```python
from build123d import *

# Parameters (mm, degrees)
BASE_FLANGE1_DEPTH            = 5
EDGE_FLANGE1_STRIP_W          = 25.2
EDGE_FLANGE1_STRIP_H          = 5
EDGE_FLANGE1_STRIP_CUT_DEPTH  = 270
EDGE_FLANGE1_RELIEF_W         = 27.7
EDGE_FLANGE1_RELIEF_H         = 2.5
EDGE_FLANGE1_RELIEF_CUT_DEPTH = 5
EDGE_FLANGE1_DEPTH            = 270
SKETCH9_R                     = 2.5
CUT_EXTRUDE1_DEPTH            = 10
FILLET1_R                     = 20
FILLET2_R                     = 2


# Sheet-metal steps are written as plain solids
with BuildPart() as part:
    # Sketch1 → Base-Flange1 (new body)
    with BuildSketch(Plane.XY):
        Polygon((28.8, 215), (-153.8, 215), (-153.8, 50), (46.2, 50), (46.2, -50), (-153.8, -50), (-153.8, -215), (28.8, -215), (28.8, -150), (153.8, -150), (153.8, 150), (28.8, 150), align=None)
    extrude(amount=-BASE_FLANGE1_DEPTH)

    # Edge-Flange1 strip (across the edge) → Edge-Flange1 strip cut (cut)
    with BuildSketch(Plane(origin=(153.8, 135, -5), x_dir=(-1, 0, 0), z_dir=(0, -1, 0))):
        with Locations((-10, -2.5)):
            Rectangle(EDGE_FLANGE1_STRIP_W, EDGE_FLANGE1_STRIP_H)
    extrude(amount=EDGE_FLANGE1_STRIP_CUT_DEPTH, mode=Mode.SUBTRACT)

    # Edge-Flange1 relief (on the sheet) → Edge-Flange1 relief cut (cut)
    with BuildSketch(Plane(origin=(151.2, 135, -5), x_dir=(-1, 0, 0), z_dir=(0, 0, -1))):
        with Locations((-11.35, 1.25)):
            Rectangle(EDGE_FLANGE1_RELIEF_W, EDGE_FLANGE1_RELIEF_H)
        with Locations((-11.35, -271.25)):
            Rectangle(EDGE_FLANGE1_RELIEF_W, EDGE_FLANGE1_RELIEF_H)
    extrude(amount=-EDGE_FLANGE1_RELIEF_CUT_DEPTH, mode=Mode.SUBTRACT)

    # Edge-Flange1 section (across the edge) → Edge-Flange1 (add)
    with BuildSketch(Plane(origin=(153.8, 135, -5), x_dir=(-1, 0, 0), z_dir=(0, -1, 0))):
        with BuildLine():
            Line((-5, 2.6), (-5, 20))
            Line((-5, 20), (0, 20))
            Line((0, 20), (0, 2.6))
            ThreePointArc((0, 2.6), (0.761522369, 0.761522369), (2.6, 0))
            Line((2.6, 0), (2.6, -5))
            ThreePointArc((2.6, -5), (-2.774011537, -2.774011537), (-5, 2.6))
        make_face()
    extrude(amount=EDGE_FLANGE1_DEPTH)

    # Sketch9 → Cut-Extrude1 (cut)
    with BuildSketch(Plane(origin=(158.8, 0, 0), x_dir=(0, 0, -1), z_dir=(1, 0, 0))):
        with Locations((17, 80)):
            Circle(SKETCH9_R)
        with Locations((17, -80)):
            Circle(SKETCH9_R)
    extrude(amount=-CUT_EXTRUDE1_DEPTH, mode=Mode.SUBTRACT)

    # Fillet1
    fillet1_edges = [part.edges().sort_by_distance(p)[0] for p in [
        (28.8, 150, -2.5),
        (28.8, -150, -2.5),
    ]]
    fillet(fillet1_edges, radius=FILLET1_R)

    # Fillet2
    fillet2_edges = [part.edges().sort_by_distance(p)[0] for p in [
        (-153.8, -50, -2.5),
        (-153.8, 50, -2.5),
        (-153.8, 215, -2.5),
        (-153.8, -215, -2.5),
    ]]
    fillet(fillet2_edges, radius=FILLET2_R)


solid = part.part
```
Geometry check sheet. Reference: the model listing, model coordinates, mm. A direction names the side the tool comes from. Coordinates: 2 decimals unless noted, no trailing zeros. Order: outer loops, then holes, each group sorted by start corner. A loop starts at its lowest first (then second) coordinate and runs counter-clockwise, first axis right, second up. Notation, with made-up numbers: (64.25, -12.75) - (108.25, -12.75) arc R24 ccw to (108.25, 4.25) - close; hole circle Ø4 at (-17.5, 23.5). An arc over 180 degrees is marked (long way). Answer as a JSON object with one key per item and string values. Group by question number.
Item 1: Sectioned sample at A-A, the plane y = 7. Record the cut outline in (x, z).
Item 2: Sectioned sample at C-C, the plane y = 94. Record the cut outline in (x, z).
Item 3: Draft check along Y on faces 4 (the face through (155, 135, -13)), 5 (the face through (-2, 51, -5)), 6 (the face through (34.814, -155.703, -2.535)). Enter one of: +Y half, -Y half, draft (parallel to the pull), parting line (faces both ways), or undercut.
Item 4: Scan lines: probe 1 along Y at (x, z) = (155.6, -17); probe 2 along Y at (x, z) = (-118, -4); probe 3 along Z at (x, y) = (20, 78). Record each from-to range of solid material in increasing order.
Item 5: Sectioned sample at B-B, the plane x = 105.5. Record the cut outline in (y, z).
Item 6: Depth check by flat-ended pin: pin 1 Ø5.5 at (x, z) = (120, -2.5) entering from +Y; pin 2 Ø3 at (x, z) = (154, -17.5) entering from -Y; pin 3 Ø4 at (y, z) = (-143.5, -3.5) entering from +X; pin 4 Ø4 at (y, z) = (-80, -17) entering from +X. Enter the tip coordinate at first touch or a pass-through.
Item 7: Tool access check on faces 1 (the face through (155, -135, -13)), 2 (the face through (153.8, 2, -16)), 3 (the face through (-2, 51, 0)). Record the directions out of +Z, -Z, +X, -X, +Y, -Y that give a thin tool (end or side, any length) a straight path to the whole face; none if there is none.
Resolved:
{
 "1": {"outline": "(46.2, -5) - (151.2, -5) arc R2.6 cw to (153.8, -7.6) - (153.8, -25) - (158.8, -25) - (158.8, -7.6) arc R7.6 ccw to (151.2, 0) - (46.2, 0) - close"},
 "2": {"outline": "(-153.8, -5) - (151.2, -5) arc R2.6 cw to (153.8, -7.6) - (153.8, -25) - (158.8, -25) - (158.8, -7.6) arc R7.6 ccw to (151.2, 0) - (-153.8, 0) - close"},
 "3": {"face 4": "undercut", "face 5": "draft", "face 6": "-Y half"},
 "4": {"probe 1": "-135 to -82.5, -77.5 to 77.5, 82.5 to 135", "probe 2": "-215 to -50, 50 to 215", "probe 3": "-5 to 0"},
 "5": {"outline": "(-150, -5) - (150, -5) - (150, 0) - (-150, 0) - close"},
 "6": {"pin 1": "y = 150", "pin 2": "y = -135", "pin 3": "x = 153.8", "pin 4": "through"},
 "7": {"face 1": "+Z, -Z, +X", "face 2": "-Z, -X, +Y, -Y", "face 3": "+Z, +X, -X, +Y, -Y"}
}
